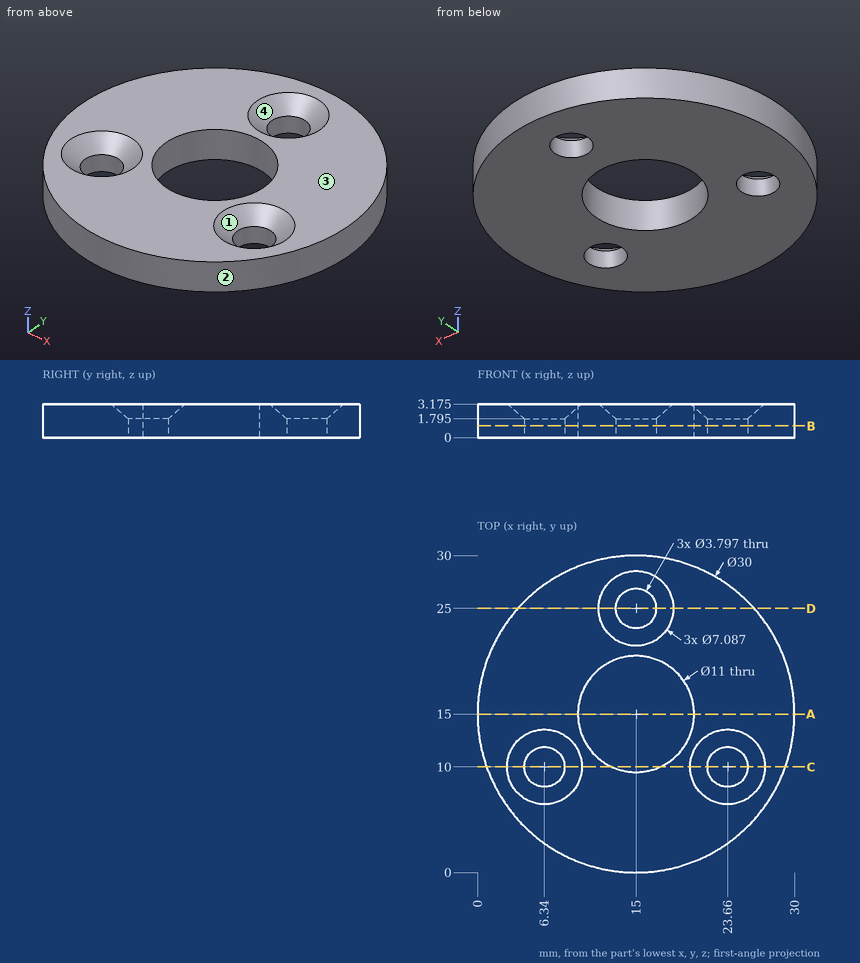
Answer from the drawing. Dimensions are ordinates in mm from the lowest x, y and z of the part. Round coordinates to 2 decimals unless told otherwise and drop trailing zeros. Order: outer loops, then holes, each group sorted by start corner. A loop starts at its lowest first (then second) coordinate and runs counter-clockwise, first axis right, second up. Notation, with made-up numbers: (21.5, 40) - (54.5, 40) arc R19 ccw to (54.5, 46) - close; hole circle Ø8 at (33, 56.5). An arc over 180 degrees is marked (long way). Put each result on its own line as item: value. Start each with the question number.
(1) Find section D-D (y = 25). Give the vertices of the cut face in (x, z) (1 decimal).
(2) Find section B-B (z = 1.1). Give the vertices of the cut face in (x, y), plus the area to 3 significant figures.
(3) Determine the mould class of the marked faces 1, 2, 3 and 4 for opening direction Y: released by +Y, released by -Y, zero draft, split by the parting line, or undercut.
(4) Straight lines are drawn through the part: probe 1 along Y at (x, z) = (15, 1.3); probe 2 along X at (y, z) = (10, 0.55) (1 decimal); probe 3 along Y at (x, z) = (15, 1.9) (1 decimal). For each, find the intervals that lie inside material, in ascending order. Write a range as from..to.
(5) Find section A-A (y = 15). Give the vertices of the cut face in (x, z) (1 decimal).
(6) Find section C-C (y = 10). Give the vertices of the cut face in (x, z) (1 decimal).
Reply:
1. outline: (3.8, 0) - (13.1, 0) - (13.1, 1.8) - (11.5, 3.2) - (3.8, 3.2) - close; (16.9, 0) - (26.2, 0) - (26.2, 3.2) - (18.5, 3.2) - (16.9, 1.8) - close
2. outline: circle Ø30 at (15, 15); hole circle Ø3.8 at (6.34, 10); hole circle Ø11 at (15, 15); hole circle Ø3.8 at (15, 25); hole circle Ø3.8 at (23.66, 10)
2. area: 578 mm^2
3. face 1: undercut
3. face 2: split by the parting line
3. face 3: zero draft
3. face 4: undercut
4. probe 1: 0..9.5, 20.5..23.1, 26.9..30
4. probe 2: 0.9..4.4, 8.2..12.7, 17.3..21.8, 25.6..29.1
4. probe 3: 0..9.5, 20.5..23, 27..30
5. outline: (0, 0) - (9.5, 0) - (9.5, 3.2) - (0, 3.2) - close; (20.5, 0) - (30, 0) - (30, 3.2) - (20.5, 3.2) - close
6. outline: (0.9, 0) - (4.4, 0) - (4.4, 1.8) - (2.8, 3.2) - (0.9, 3.2) - close; (8.2, 0) - (12.7, 0) - (12.7, 3.2) - (9.9, 3.2) - (8.2, 1.8) - close; (17.3, 0) - (21.8, 0) - (21.8, 1.8) - (20.1, 3.2) - (17.3, 3.2) - close; (25.6, 0) - (29.1, 0) - (29.1, 3.2) - (27.2, 3.2) - (25.6, 1.8) - close
